```python
from build123d import *

# Parameters (mm, degrees)
SKETCH1_W           = 200
SKETCH1_H           = 40
BOSS_EXTRUDE1_DEPTH = 3
SKETCH3_W           = 60
SKETCH3_H           = 3
SKETCH3_W_2         = 60.649381746
CUT_EXTRUDE1_DEPTH  = 3
SKETCH4_R           = 1.5
CUT_EXTRUDE2_DEPTH  = 3


with BuildPart() as part:
    # Sketch1 → Boss-Extrude1 (new body)
    with BuildSketch(Plane(origin=(0, 0, 0), x_dir=(1, 0, 0), z_dir=(0, 1, 0))):
        Rectangle(SKETCH1_W, SKETCH1_H)
    extrude(amount=BOSS_EXTRUDE1_DEPTH)

    # Sketch3 → Cut-Extrude1 (cut)
    with BuildSketch(Plane(origin=(0, 3, 0), x_dir=(1, 0, 0), z_dir=(0, 1, 0))):
        Polygon((-20, -20), (-20, -17), (-1.5, -17), (-1.5, -15), (-2.75, -15), (-2.75, -12), (-1.5, -12), (-1.5, -10), (1.5, -10), (1.5, -12), (2.75, -12), (2.75, -15), (1.5, -15), (1.5, -17), (20, -17), (20, -20), align=None)
        with Locations((-70, -18.5)):
            Rectangle(SKETCH3_W, SKETCH3_H)
        with Locations((69.675309127, -18.5)):
            Rectangle(SKETCH3_W_2, SKETCH3_H)
        Polygon((85, 17), (100, 17), (100, 20), (60, 20), (60, 17), (82, 17), align=None)
        Polygon((20, 20), (20, 17), (1.5, 17), (1.5, 15), (2.75, 15), (2.75, 12), (1.5, 12), (1.5, 10), (-1.5, 10), (-1.5, 12), (-2.75, 12), (-2.75, 15), (-1.5, 15), (-1.5, 17), (-20, 17), (-20, 20), align=None)
        Polygon((-60, 20), (-60, 17), (-82, 17), (-85, 17), (-100, 17), (-100, 20), align=None)
    extrude(amount=-CUT_EXTRUDE1_DEPTH, mode=Mode.SUBTRACT)

    # Sketch4 → Cut-Extrude2 (cut)
    with BuildSketch(Plane(origin=(0, 3, 0), x_dir=(1, 0, 0), z_dir=(0, 1, 0))):
        with Locations(Location((92.5, 14.5, 0), (0, 0, 270))):
            Circle(SKETCH4_R)
        with Locations(Location((-77.5, 14.5, 0), (0, 0, 270))):
            Circle(SKETCH4_R)
    extrude(amount=-CUT_EXTRUDE2_DEPTH, mode=Mode.SUBTRACT)


solid = part.part
```
Could you check a few things on this model? Use its own coordinates, in mm. Round coordinates to 2 decimals unless told otherwise and drop trailing zeros. Write each loop counter-clockwise with the first axis right and the second up, starting at its lowest first coordinate (ties: lowest second). Pieces come first, ordered by that corner, then holes.
(1) Suppose I cut it at B-B on y = 0.6. State how many separate pieces and enclosed holes the cut face has, and give its area (3 significant figures).
Findings below:
separate pieces: 1
enclosed holes: 2
area: 7,090 mm2
(2) Suppose I cut it at A-A on x = 71.5. Write out the boundary of the cut face in (y, z), and give its area (3 significant figures).
Findings below:
outline: (0, -17) - (3, -17) - (3, 17) - (0, 17) - close
area: 102 mm2
(3) For pin 1 (3.5 mm diameter, centred on x = 92.5, z = -14.5, fed in from -Y); pin 2 (1 mm diameter, centred on x = -2, y = 2, fed in from +Z); pin 3 (0.9 mm diameter, centred on x = 10, y = 1.5, fed in from -Z); pin 4 (1.5 mm diameter, centred on y = 1, z = 18, fed in from +X), each with a flat end and sliding along its axis, tell me the tip position at first contact or that it passes through.
Findings below:
pin 1: stops at y = 0
pin 2: stops at z = 17
pin 3: stops at z = -17
pin 4: stops at x = 39.35
(4) If I drill on probe 1 along X at (y, z) = (1.25, -14.5); probe 2 along Z at (x, y) = (-77.5, 2.05); probe 3 along X at (y, z) = (0.35, -13.5), over which ranges is the centre line in solid material (lowest first)?
Findings below:
probe 1: x = -100 to -79, -76 to -2.75, 2.75 to 91, 94 to 100
probe 2: z = -17 to -16, -13 to 17
probe 3: x = -100 to -78.62, -76.38 to -2.75, 2.75 to 91.38, 93.62 to 100
